Here's how the part is built. I have some questions about the finished solid (model axes, mm). Face numbers are marked on the shaded views. A direction names the side the tool comes from. Give positions to 0.01 mm unless a question says otherwise; leave off trailing zeros. Order: outer loops, then holes, each group sorted by start corner. A loop starts at its lowest first (then second) coordinate and runs counter-clockwise, first axis right, second up. Notation, with made-up numbers: M -6.75,-15.75 L 39.25,-15.75 A27 ccw 39.25,15.25 Z; hole C 65,10 d4. An arc over 180 degrees is marked long. Use one line per item in the form item = value.
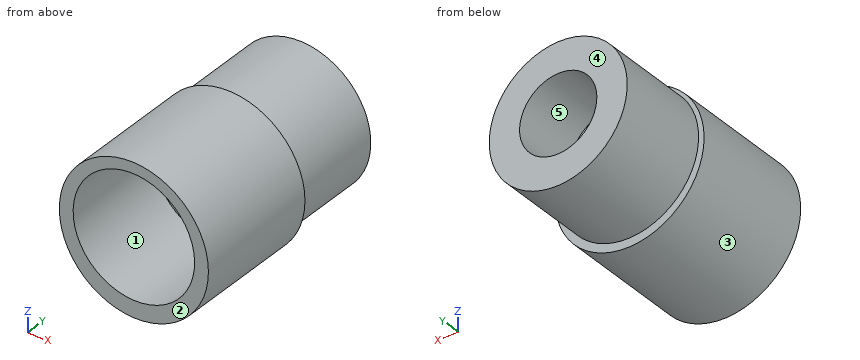
from build123d import *

# Parameters (mm, degrees)
SKETCH1_R           = 3.175
BOSS_EXTRUDE1_DEPTH = 4.318
SKETCH2_R           = 1.778
CUT_EXTRUDE1_DEPTH  = 3.048
SKETCH4_R           = 3.429
BOSS_EXTRUDE2_DEPTH = 5.842
SKETCH5_R           = 2.794
CUT_EXTRUDE2_DEPTH  = 4.826


with BuildPart() as part:
    # Sketch1 → Boss-Extrude1 (new body)
    with BuildSketch(Plane(origin=(0, 0, 0), x_dir=(1, 0, 0), z_dir=(0, 1, 0))):
        with Locations(Location((0, 0, 0), (0, 0, 270))):
            Circle(SKETCH1_R)
    extrude(amount=BOSS_EXTRUDE1_DEPTH)

    # Sketch2 → Cut-Extrude1 (cut)
    with BuildSketch(Plane(origin=(0, 4.318, 0), x_dir=(1, 0, 0), z_dir=(0, 1, 0))):
        with Locations(Location((0, 0, 0), (0, 0, 270))):
            Circle(SKETCH2_R)
    extrude(amount=-CUT_EXTRUDE1_DEPTH, mode=Mode.SUBTRACT)

    # Sketch4 → Boss-Extrude2 (add)
    with BuildSketch(Plane.XZ):
        with Locations(Location((0, -0.136069794, 0), (0, 0, 270))):
            Circle(SKETCH4_R)
    extrude(amount=BOSS_EXTRUDE2_DEPTH)

    # Sketch5 → Cut-Extrude2 (cut)
    with BuildSketch(Plane.XZ.offset(5.842)):
        with Locations(Location((0, 0, 0), (0, 0, 270))):
            Circle(SKETCH5_R)
    extrude(amount=-CUT_EXTRUDE2_DEPTH, mode=Mode.SUBTRACT)


solid = part.part
Q1. I need wall thicknesses on L1, parallel to X at y = -4.2, z = 0; L2, parallel to X at y = 3.05, z = 0 (3 decimals); L3, parallel to Y at x = 2.5, z = 2. Which ranges of each line are inside material? Lowest first, please.
Found:
L1 = -3.43 to -2.79, 2.79 to 3.43
L2 = -3.175 to -1.778, 1.778 to 3.175
L3 = -5.84 to 0
Q2. I want a section at A-A on x = 0. Write out the boundary of the cut face in (y, z) (3 decimals), then the cut area to 3 significant figures.
Found:
outline = M -5.842,-3.565 L 0,-3.565 L 0,-3.175 L 4.318,-3.175 L 4.318,-1.778 L 1.27,-1.778 L 1.27,1.778 L 4.318,1.778 L 4.318,3.175 L 0,3.175 L 0,3.293 L -5.842,3.293 L -5.842,2.794 L -1.016,2.794 L -1.016,-2.794 L -5.842,-2.794 Z
area = 29.7 mm²
Q3. I'm going to push flat-ended pins straight in: pin 1 Ø1.1 at (x, z) = (1, -1) entering from +Y; pin 2 Ø1.5 at (x, y) = (-1.5, 2.5) entering from -Z; pin 3 Ø1.5 at (y, z) = (-2, 1) entering from -X; pin 4 Ø2 at (x, z) = (0, 0) entering from -Y. Where does each tip first touch, or does it pass through?
Found:
pin_1 = 4.32
pin_2 = -3.09
pin_3 = -3.41
pin_4 = -1.02
Q4. I want a section at B-B on z = -1. Write out the boundary of the cut face in (x, y), then the cut area to 3 significant figures.
Found:
outline = M -3.32,-5.84 L -2.61,-5.84 L -2.61,-1.02 L 2.61,-1.02 L 2.61,-5.84 L 3.32,-5.84 L 3.32,0 L 3.01,0 L 3.01,4.32 L 1.47,4.32 L 1.47,1.27 L -1.47,1.27 L -1.47,4.32 L -3.01,4.32 L -3.01,0 L -3.32,0 Z
area = 30.7 mm²
Q5. I want a section at D-D on x = -2. Write out the boundary of the cut face in (y, z).
Found:
outline = M -5.84,-2.92 L 0,-2.92 L 0,-2.47 L 4.32,-2.47 L 4.32,2.47 L 0,2.47 L 0,2.65 L -5.84,2.65 L -5.84,1.95 L -1.02,1.95 L -1.02,-1.95 L -5.84,-1.95 Z
Q6. I want a section at C-C on y = -1.25. Write out the boundary of the cut face in (x, z), then the cut area to 3 significant figures.
Found:
outline = C 0,-0.14 d6.86; hole C 0,0 d5.59
area = 12.4 mm²
Q7. Thinking about a two-plate mould opening in X: for the marked faces 1, 2 and 3, which applies, +X half, -X half, draft (parallel to the pull), parting line (faces both ways), or undercut?
Found:
face_1 = undercut
face_2 = draft
face_3 = parting line
Q8. On a 3-axis mill with a long thin cutter (end or side, diameter ignored), from which of +Z, -Z, +X, -X, +Y, -Y can I reach the whole of each face in a straight line? I mean the marked faces 4 and 5. Say none if no direction works.
Found:
face_4 = +Z, -Z, +X, -X, +Y
face_5 = +Y
